Here's how the part is built. I have some questions about the finished solid (model axes, mm). Face numbers are marked on the shaded views. A direction names the side the tool comes from. Coordinates: 2 decimals unless noted, no trailing zeros. Loops run counter-clockwise (first coordinate to the right, second up) from the corner with the lowest first, then second, coordinate; pieces in that order, holes last. Notation, with made-up numbers: M -13.75,14.5 L 28.25,14.5 A17 ccw 28.25,21.5 Z; hole C 16,-4 d11. An arc over 180 degrees is marked long. Use one line per item in the form item = value. Start each with the question number.
(1) Imagine slicing it at C-C, the plane z = -4.5. Please give me the cut outline in (x, y).
(2) Thinking about a two-plate mould opening in Y: for the marked faces 1, 2 and 3, which applies, +Y half, -Y half, draft (parallel to the pull), parting line (faces both ways), or undercut?
(3) Please list where these lines run through material, in increasing order: L1, parallel to X at y = -8.5, z = -13; L2, parallel to Y at x = -34.5, z = -3.75; L3, parallel to Z at x = -1, y = -9.
(4) Imagine slicing it at B-B, the plane x = -25. Please give me the cut outline in (y, z), and give its area (3 significant figures).
(5) On a 3-axis mill with a long thin cutter (end or side, diameter ignored), from which of +Z, -Z, +X, -X, +Y, -Y can I reach the whole of each face in a straight line? I mean the marked faces 4 and 5. Say none if no direction works.
(6) Imagine slicing it at A-A, the plane z = -8.5. Please give me the cut outline in (x, y).
(7) Will these pins go through, and if not, where does the flat tip stop? P1, Ø1.6, axis at x = -25, y = -34.5, coming from the +Z side; P2, Ø17, axis at x = -16, y = 5, coming from the -Z side; P3, Ø1.6, axis at x = 49.5, y = -4, coming from the -Z side; P4, Ø5.5, axis at x = 33.67, y = -5.89, coming from the -Z side.
(8) Imagine slicing it at D-D, the plane x = 29. Please give me the cut outline in (y, z).
```python
from build123d import *

# Parameters (mm, degrees)
ESQUISSE1_W             = 89
ESQUISSE1_H             = 57
BOSS_EXTRU_1_DEPTH      = 2
ESQUISSE2_W             = 16
ESQUISSE2_H             = 57
BOSS_EXTRU_2_DEPTH      = 2
ESQUISSE3_W             = 16
ESQUISSE3_H             = 57
BOSS_EXTRU_3_DEPTH      = 2
ESQUISSE4_W             = 93
ESQUISSE4_H             = 16
BOSS_EXTRU_4_DEPTH      = 2
ESQUISSE5_W             = 93
ESQUISSE5_H             = 16
BOSS_EXTRU_5_DEPTH      = 2
ESQUISSE6_R             = 3
ENL_V_MAT_EXTRU_1_DEPTH = 2
ESQUISSE7_R             = 3
ENL_V_MAT_EXTRU_2_DEPTH = 2
ESQUISSE11_W            = 5
ESQUISSE11_H            = 10
ENL_V_MAT_EXTRU_3_DEPTH = 2
ESQUISSE13_W            = 2.999998882
ESQUISSE13_H            = 5
ENL_V_MAT_EXTRU_4_DEPTH = 2
ESQUISSE14_W            = 9
ESQUISSE14_H            = 4
ENL_V_MAT_EXTRU_7_DEPTH = 2


with BuildPart() as part:
    # Esquisse1 → Boss.-Extru.1 (new body)
    with BuildSketch(Plane.XY):
        with Locations((4.166807432, -5.391891892)):
            Rectangle(ESQUISSE1_W, ESQUISSE1_H)
    extrude(amount=BOSS_EXTRU_1_DEPTH)

    # Esquisse2 → Boss.-Extru.2 (add)
    with BuildSketch(Plane(origin=(48.666807432, 0, 0), x_dir=(0, 0, -1), z_dir=(1, 0, 0))):
        with Locations((6, -5.391891892)):
            Rectangle(ESQUISSE2_W, ESQUISSE2_H)
    extrude(amount=BOSS_EXTRU_2_DEPTH)

    # Esquisse3 → Boss.-Extru.3 (add)
    with BuildSketch(Plane.ZY.offset(40.333192568)):
        with Locations((-6, -5.391891892)):
            Rectangle(ESQUISSE3_W, ESQUISSE3_H)
    extrude(amount=BOSS_EXTRU_3_DEPTH)

    # Esquisse4 → Boss.-Extru.4 (add)
    with BuildSketch(Plane.XZ.offset(33.891891892)):
        with Locations((4.166807432, -6)):
            Rectangle(ESQUISSE4_W, ESQUISSE4_H)
    extrude(amount=BOSS_EXTRU_4_DEPTH)

    # Esquisse5 → Boss.-Extru.5 (add)
    with BuildSketch(Plane(origin=(0, 23.108108108, 0), x_dir=(1, 0, 0), z_dir=(0, 1, 0))):
        with Locations((4.166807432, 6)):
            Rectangle(ESQUISSE5_W, ESQUISSE5_H)
    extrude(amount=BOSS_EXTRU_5_DEPTH)

    # Esquisse6 → Enlèv. mat.-Extru.1 (cut)
    with BuildSketch(Plane(origin=(0, 0, 0), x_dir=(-1, 0, 0), z_dir=(0, 0, -1))):
        with Locations((25.333192568, -5.891891892)):
            Circle(ESQUISSE6_R)
    extrude(amount=-ENL_V_MAT_EXTRU_1_DEPTH, mode=Mode.SUBTRACT)

    # Esquisse7 → Enlèv. mat.-Extru.2 (cut)
    with BuildSketch(Plane(origin=(0, 0, 0), x_dir=(-1, 0, 0), z_dir=(0, 0, -1))):
        with Locations((-33.666807432, -5.891891892)):
            Circle(ESQUISSE7_R)
    extrude(amount=-ENL_V_MAT_EXTRU_2_DEPTH, mode=Mode.SUBTRACT)

    # Esquisse11 → Enlèv. mat.-Extru.3 (cut)
    with BuildSketch(Plane(origin=(50.666807432, 0, 0), x_dir=(0, 0, -1), z_dir=(1, 0, 0))):
        with Locations((8.500001118, -5.394481666)):
            Rectangle(ESQUISSE11_W, ESQUISSE11_H)
    extrude(amount=-ENL_V_MAT_EXTRU_3_DEPTH, mode=Mode.SUBTRACT)

    # Esquisse13 → Enlèv. mat.-Extru.4 (cut)
    with BuildSketch(Plane(origin=(50.666807432, 0, 0), x_dir=(0, 0, -1), z_dir=(1, 0, 0))):
        with Locations((12.500000559, -5.394481666)):
            Rectangle(ESQUISSE13_W, ESQUISSE13_H)
    extrude(amount=-ENL_V_MAT_EXTRU_4_DEPTH, mode=Mode.SUBTRACT)

    # Esquisse14 → Enlèv. mat.-Extru.7 (cut)
    with BuildSketch(Plane.XY.offset(2)):
        with Locations((-26.833192568, -33.891891892)):
            Rectangle(ESQUISSE14_W, ESQUISSE14_H)
    extrude(amount=-ENL_V_MAT_EXTRU_7_DEPTH, mode=Mode.SUBTRACT)


solid = part.part
```
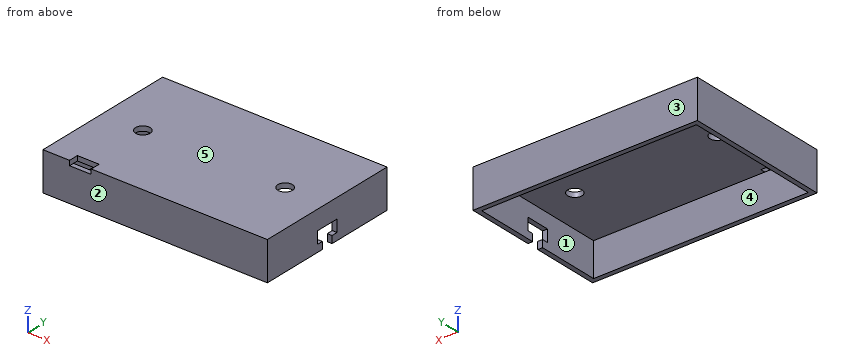
Answer:
q1.outline = M -42.33,-35.89 L 50.67,-35.89 L 50.67,25.11 L -42.33,25.11 Z; hole M -40.33,-33.89 L 48.67,-33.89 L 48.67,23.11 L -40.33,23.11 Z
q2.face_1 = undercut
q2.face_2 = -Y half
q2.face_3 = +Y half
q3.L1 = -42.33 to -40.33, 48.67 to 50.67
q3.L2 = -35.89 to -33.89, 23.11 to 25.11
q3.L3 = 0 to 2
q4.outline = M -35.89,-14 L -33.89,-14 L -33.89,0 L -35.89,0 Z; M -31.89,0 L -8.87,0 L -8.87,2 L -31.89,2 Z; M -2.91,0 L 23.11,0 L 23.11,-14 L 25.11,-14 L 25.11,2 L -2.91,2 Z
q4.area = 158 mm²
q5.face_4 = -Z
q5.face_5 = +Z, +X, -X, +Y, -Y
q6.outline = M -42.33,-35.89 L 50.67,-35.89 L 50.67,-10.39 L 48.67,-10.39 L 48.67,-33.89 L -40.33,-33.89 L -40.33,23.11 L 48.67,23.11 L 48.67,-0.39 L 50.67,-0.39 L 50.67,25.11 L -42.33,25.11 Z
q7.P1 = 0
q7.P2 = 0
q7.P3 = -6
q7.P4 = through
q8.outline = M -35.89,-14 L -33.89,-14 L -33.89,0 L 23.11,0 L 23.11,-14 L 25.11,-14 L 25.11,2 L -35.89,2 Z
